Autodesk Inventor part; units mm, degrees
ref_plane "YZ Plane" through (0, 0, 0) normal (1, 0, 0) x (0, 1, 0)
ref_plane "XZ Plane" through (0, 0, 0) normal (0, 1, 0) x (-1, 0, 0)
ref_plane "XY Plane" through (0, 0, 0) normal (0, 0, 1) x (1, 0, 0)
sketch "Sketch1" plane through (0, 0, 0) normal (0, 0, 1) x (1, 0, 0)
  circle A0 centre (0, 0) radius 100
  circle A1 centre (0, 0) radius 157.5
  dimension "d22" = 200
  dimension "d23" = 315
extrude "Plate1" add sketch "Sketch1" along normal blind 10
sketch "Sketch5" plane through (0, 0, 10) normal (0, 0, 1) x (1, 0, 0)
  circle A0 centre (0, 140) radius 11
  circle A1 centre (0, 0) radius 140 construction
  dimension "d25" = 280
  dimension "d24" = 22
extrude "Cut1" cut sketch "Sketch5" against normal blind 10
pattern_circular "Circular Pattern1" count 8 over 360 about axis through (0, 0, 0) along (0, 0, 1) of "Cut1"
equation "\"d26\" = Thickness"
equation "\"d2\" = Thickness"
equation "\"BendReliefDepth\" = 0.5 * Thickness"
equation "\"TransitionRadius\" = BendRadius"
equation "\"JacobiRadiusSize\" = BendRadius"
properties part number "Main filter Flange" material "Stainless Steel"
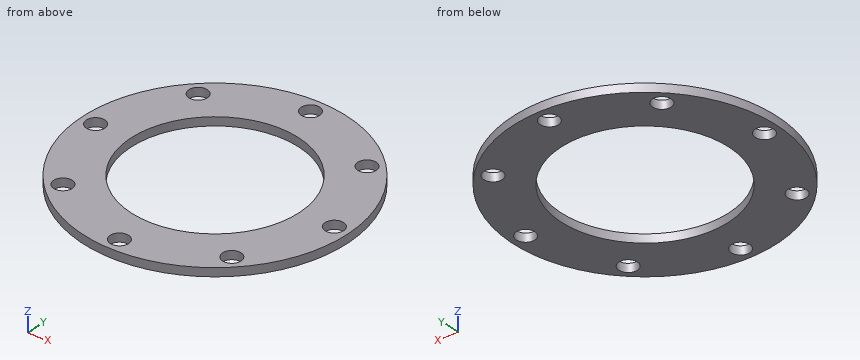
CAD build for the part. Positions are in the model's coordinates, mm. Round coordinates to 2 decimals unless told otherwise and drop trailing zeros. Order: outer loops, then holes, each group sorted by start corner. A loop starts at its lowest first (then second) coordinate and runs counter-clockwise, first axis right, second up. Notation, with made-up numbers: (53, 62.25) - (96, 62.25) arc R14 ccw to (96, 87.25) - close; hole circle Ø7 at (79, -23). An arc over 180 degrees is marked (long way). Answer in a Markdown table with one row per item. Add a question column.
(1) Band-saw the part on D-D on z = 1.5. Count the separate pieces of the cut face and the enclosed holes in it, and give its area (3 significant figures).
(2) Band-saw the part on A-A on x = 0. List the corners of the cut face in (y, z), and give its area (3 significant figures).
(3) Probe L1, parallel to Y at x = 0, z = 7.75; L2, parallel to X at y = -6.5, z = 5.5; L3, parallel to X at y = 85, z = 5.25. List the from-to ranges inside material, lowest first. Write a range as [from, to].
(4) Band-saw the part on C-C on x = 140. List the corners of the cut face in (y, z).
(5) Drop flat-ended pins along their axis: pin 1 Ø4 at (y, z) = (-95, 4) entering from -X; pin 2 Ø1 at (x, z) = (46, 2.5) entering from +Y; pin 3 Ø6 at (x, z) = (82.5, 6.5) entering from -Y. Give the stop position or say it passes through.
Data:
| question | item | result |
|---|---|---|
| 1 | separate pieces | 1 |
| 1 | enclosed holes | 9 |
| 1 | area | 43,500 mm^2 |
| 2 | outline | (-157.5, 0) - (-151, 0) - (-151, 10) - (-157.5, 10) - close; (-129, 0) - (-100, 0) - (-100, 10) - (-129, 10) - close; (100, 0) - (129, 0) - (129, 10) - (100, 10) - close; (151, 0) - (157.5, 0) - (157.5, 10) - (151, 10) - close |
| 2 | area | 710 mm^2 |
| 3 | L1 | y = [-157.5, -151], [-129, -100], [100, 129], [151, 157.5] |
| 3 | L2 | x = [-157.37, -148.87], [-131.13, -99.79], [99.79, 131.13], [148.87, 157.37] |
| 3 | L3 | x = [-132.59, -52.68], [52.68, 132.59] |
| 4 | outline | (-72.15, 0) - (-11, 0) - (-11, 10) - (-72.15, 10) - close; (11, 0) - (72.15, 0) - (72.15, 10) - (11, 10) - close |
| 5 | pin 1 | stops at x = -127.11 |
| 5 | pin 2 | stops at y = 150.78 |
| 5 | pin 3 | stops at y = -135.96 |
